Verification items for the finished model (mm, model axes). Face numbers are marked on the shaded views. Round coordinates to 2 decimals unless told otherwise and drop trailing zeros. Loops run counter-clockwise (first coordinate to the right, second up) from the corner with the lowest first, then second, coordinate; pieces in that order, holes last. Notation, with made-up numbers: M 36.5,38 L 89.5,38 A32 ccw 89.5,75 Z; hole C -19,35 d1. An arc over 180 degrees is marked long. Answer as CSV lines item,"result".
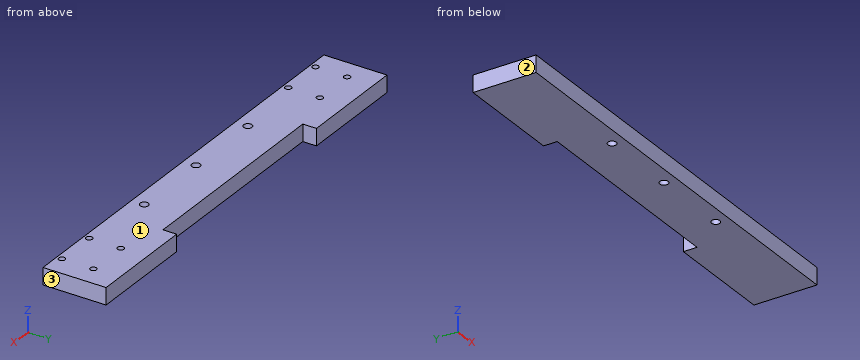
```python
from build123d import *

# Parameters (mm, degrees)
BOSS_EXTRU_1_DEPTH      = 8
ESQUISSE2_R             = 2
ENL_V_MAT_EXTRU_1_DEPTH = 9
ESQUISSE3_R             = 1.5
ENL_V_MAT_EXTRU_2_DEPTH = 5


with BuildPart() as part:
    # Esquisse1 → Boss.-Extru.1 (new body)
    with BuildSketch(Plane.XY):
        Polygon((0, 30), (0, 0), (206, 0), (206, 30), (154.25, 30), (154.25, 23.5), (51.75, 23.5), (51.75, 30), align=None)
    extrude(amount=BOSS_EXTRU_1_DEPTH)

    # Esquisse2 → Enlèv. mat.-Extru.1 (cut, through all)
    with BuildSketch(Plane.XY.offset(8)):
        with Locations((103, 6)):
            Circle(ESQUISSE2_R)
        with Locations((141, 6)):
            Circle(ESQUISSE2_R)
        with Locations((65, 6)):
            Circle(ESQUISSE2_R)
    extrude(amount=-ENL_V_MAT_EXTRU_1_DEPTH, mode=Mode.SUBTRACT)

    # Esquisse3 → Enlèv. mat.-Extru.2 (cut)
    with BuildSketch(Plane.XY.offset(8)):
        with Locations((176, 17.5)):
            Circle(ESQUISSE3_R)
        with Locations((196, 17.5)):
            Circle(ESQUISSE3_R)
        with Locations((196, 2.5)):
            Circle(ESQUISSE3_R)
        with Locations((176, 2.5)):
            Circle(ESQUISSE3_R)
    enl_v_mat_extru_2 = extrude(amount=-ENL_V_MAT_EXTRU_2_DEPTH, mode=Mode.SUBTRACT)

    # Symétrie1: Enlèv. mat.-Extru.2 across plane
    add(enl_v_mat_extru_2.mirror(Plane(origin=(103, 0, 0), x_dir=(0, 0, 1), z_dir=(1, 0, 0))), mode=Mode.SUBTRACT)


solid = part.part
```
1) Go/stop test with flat-tipped pins: pin 1 (2.5 mm diameter, centred on x = 10, y = 17.5, fed in from +Z); pin 2 (4 mm diameter, centred on x = 124.5, z = 5, fed in from +Y). Record where each tip stops, or that it passes through.
Here are the results:
pin 1,"stops at z = 3"
pin 2,"stops at y = 23.5"
2) Section check B-B (z = 1.75). Record the cut outline in (x, y).
Here are the results:
outline,"M 0,0 L 206,0 L 206,30 L 154.25,30 L 154.25,23.5 L 51.75,23.5 L 51.75,30 L 0,30 Z; hole C 65,6 d4; hole C 103,6 d4; hole C 141,6 d4"
3) Draft check along X on the marked faces 1, 2 and 3. Enter one of: +X half, -X half, draft (parallel to the pull), parting line (faces both ways), or undercut.
Here are the results:
face 1,"draft"
face 2,"-X half"
face 3,"+X half"
4) Section check C-C (x = 65). Record the cut outline in (y, z).
Here are the results:
outline,"M 0,0 L 4,0 L 4,8 L 0,8 Z; M 8,0 L 23.5,0 L 23.5,8 L 8,8 Z"
5) Material ranges on probe 1 along Y at (x, z) = (176, 4.3); probe 2 along X at (y, z) = (5, 6); probe 3 along Y at (x, z) = (144, 3.5), recorded low to high.
Here are the results:
probe 1,"y = 0 to 1, 4 to 16, 19 to 30"
probe 2,"x = 0 to 63.27, 66.73 to 101.27, 104.73 to 139.27, 142.73 to 206"
probe 3,"y = 0 to 23.5"
6) Section check A-A (y = 6). Record the cut outline in (x, z).
Here are the results:
outline,"M 0,0 L 63,0 L 63,8 L 0,8 Z; M 67,0 L 101,0 L 101,8 L 67,8 Z; M 105,0 L 139,0 L 139,8 L 105,8 Z; M 143,0 L 206,0 L 206,8 L 143,8 Z"
